from build123d import *

# Parameters (mm, degrees)
SKETCH1_R           = 10
BOSS_EXTRUDE1_DEPTH = 5
CHAMFER1_SIZE       = 2
SKETCH2_R           = 1.5
CUT_EXTRUDE1_DEPTH  = 5


with BuildPart() as part:
    # Sketch1 → Boss-Extrude1 (new body)
    with BuildSketch(Plane.XY):
        Circle(SKETCH1_R)
    extrude(amount=BOSS_EXTRUDE1_DEPTH)

    # Chamfer1
    chamfer1_edges = [part.edges().sort_by_distance(p)[0] for p in [
        (-10, 0, 5),
    ]]
    chamfer(chamfer1_edges, length=CHAMFER1_SIZE)

    # Sketch2 → Cut-Extrude1 (cut)
    with BuildSketch(Plane.XY.offset(5)):
        Circle(SKETCH2_R)
    extrude(amount=-CUT_EXTRUDE1_DEPTH, mode=Mode.SUBTRACT)


solid = part.part
The listing builds one solid part. Answer for the finished solid, in the listing's coordinates (mm). Coordinates: 2 decimals unless noted, no trailing zeros. Loops run counter-clockwise (first coordinate to the right, second up) from the corner with the lowest first, then second, coordinate; pieces in that order, holes last. Notation, with made-up numbers: (39.25, 89.5) -> (85.25, 89.5) arc R21 ccw to (85.25, 99.5) -> close; hole circle Ø10 at (13, -19.75). An arc over 180 degrees is marked (long way). Answer in a Markdown table with one row per item. Add a question column.
1. The part is cut by section D-D, the plane z = 1.75. Write down the section's boundary in (x, y), then the cut area to 3 significant figures.
2. Flat-ended cylindrical pins translate along their axes: P1, Ø3, axis at x = -5.5, z = 2, coming from the -Y side; P2, Ø8, axis at x = -7.5, y = 1.5, coming from the -Z side; P3, Ø1, axis at x = -1.5, z = 2, coming from the -Y side; P4, Ø2.5, axis at x = 0, y = 0, coming from the +Z side. Find the tip coordinate at first contact, or state that the pin passes through.
3. Determine the mould class of faces 1 (the cylindrical face through (-1.5, 0.07, 2.54)), 2 (the flat face through (2, 0, 0)), 3 (the cylindrical face through (-2.17, -9.76, 1.48)) for opening direction Y: +Y half, -Y half, draft (parallel to the pull), parting line (faces both ways), or undercut.
4. The part is cut by section A-A, the plane x = 0. Write down the section's boundary in (y, z), then the cut area to 3 significant figures.
5. The part is cut by section C-C, the plane z = 4. Write down the section's boundary in (x, y), then the cut area to 3 significant figures.
6. Consider line 1 (Y direction, x = 0, z = 2.2); line 2 (Y direction, x = -0.75, z = 3.2); line 3 (X direction, y = -0.5, z = 1.2). Determine where each line is inside the solid, lowest interval first. Write a range as [from, to].
Answer below:
| question | item | result |
|---|---|---|
| 1 | outline | circle Ø20 at (0, 0); hole circle Ø3 at (0, 0) |
| 1 | area | 307 mm2 |
| 2 | P1 | y = -9.17 |
| 2 | P2 | z = 0 |
| 2 | P3 | y = -9.95 |
| 2 | P4 | through |
| 3 | face 1 | undercut |
| 3 | face 2 | draft |
| 3 | face 3 | parting line |
| 4 | outline | (-10, 0) -> (-1.5, 0) -> (-1.5, 5) -> (-8, 5) -> (-10, 3) -> close; (1.5, 0) -> (10, 0) -> (10, 3) -> (8, 5) -> (1.5, 5) -> close |
| 4 | area | 81.0 mm2 |
| 5 | outline | circle Ø18 at (0, 0); hole circle Ø3 at (0, 0) |
| 5 | area | 247 mm2 |
| 6 | line 1 | [-10, -1.5], [1.5, 10] |
| 6 | line 2 | [-9.77, -1.3], [1.3, 9.77] |
| 6 | line 3 | [-9.99, -1.41], [1.41, 9.99] |
